Job drawing, mm, ordinate dimensions from the low corner. One solid piece. Give positions to 0.01 mm unless a question says otherwise; leave off trailing zeros. Loops run counter-clockwise (first coordinate to the right, second up) from the corner with the lowest first, then second, coordinate; pieces in that order, holes last. Notation, with made-up numbers: (15.5, 28) - (66.5, 28) arc R21 ccw to (66.5, 36) - close; hole circle Ø8 at (39.25, 80.5). An arc over 180 degrees is marked (long way). Answer as CSV lines item,"result". Start each with the question number.
Item 1: Saw through at D-D on z = 1.75. Give the cut face in (x, y), plus the area to 3 significant figures.
Item 2: Saw through at A-A on z = 9. Give the cut face in (x, y).
Item 3: Saw through at B-B on y = 1.65. State how many separate pieces and enclosed holes the cut face has, plus the area to 3 significant figures.
Item 4: Pull direction X, two halves, no side cores. Call the marked faces 1, 2 and 3: pulls with the +X half, pulls with the -X half, needs draft (parallel to the pull), parting line crosses it, or undercut.
Item 5: Pin check, flat tips, straight feed: pin 1 (1.4 mm diameter, centred on x = 5.47, z = 4.15, fed in from -Y); pin 2 (1 mm diameter, centred on x = 10, y = 0.5, fed in from -Z); pin 3 (1 mm diameter, centred on y = 1, z = 10, fed in from +X). Stop position of each tip, or through.
Item 6: Drill centre lines: L1, parallel to Z at x = 10.5, y = 0.25 (1 decimal); L2, parallel to Z at x = 4, y = 0.4 (1 decimal); L3, parallel to Z at x = 9.25, y = 0.7 (1 decimal). Where is each one in solid material? Low to high. Write a range as from..to.
Item 7: Saw through at C-C on z = 15. Give the cut face in (x, y), plus the area to 3 significant figures.
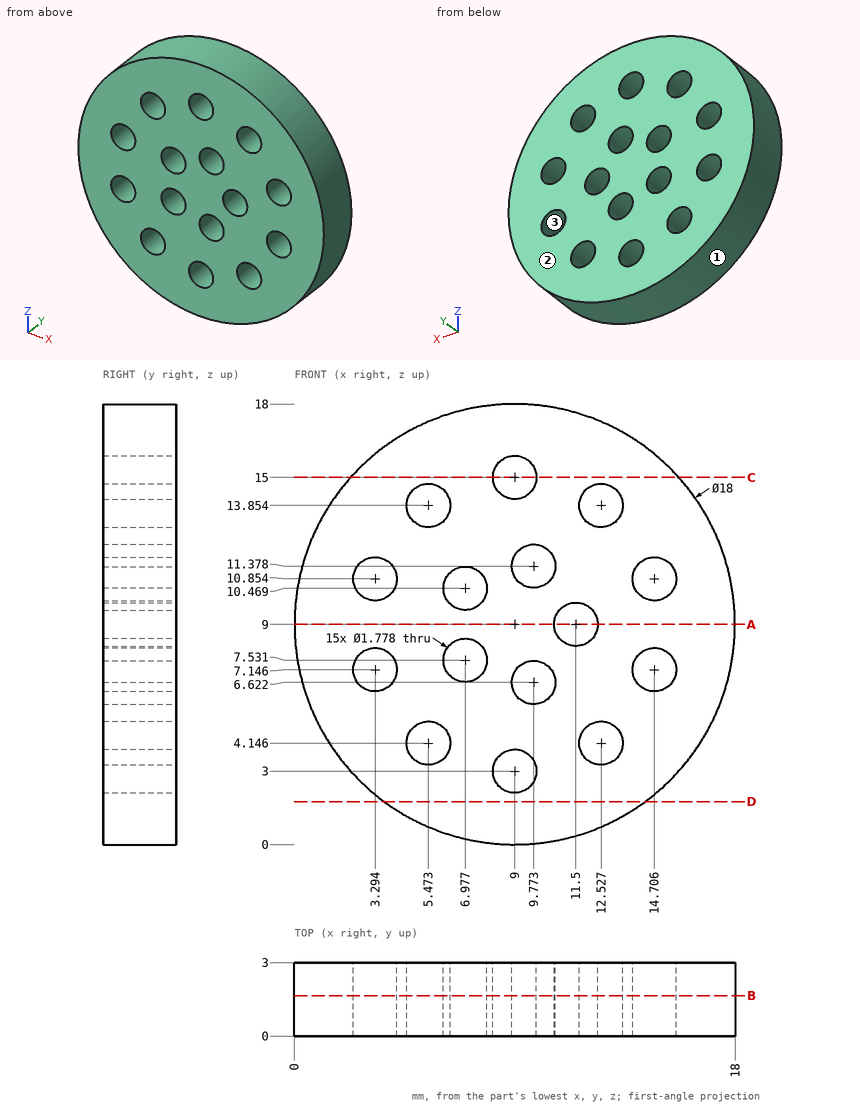
Responses:
1,outline,"(3.67, 0) - (14.33, 0) - (14.33, 3) - (3.67, 3) - close"
1,area,"32.0 mm2"
2,outline,"(0, 0) - (10.61, 0) - (10.61, 3) - (0, 3) - close; (12.39, 0) - (18, 0) - (18, 3) - (12.39, 3) - close"
3,separate pieces,"1"
3,enclosed holes,"15"
3,area,"217 mm2"
4,face 1,"parting line crosses it"
4,face 2,"needs draft"
4,face 3,"undercut"
5,pin 1,"through"
5,pin 2,"z = 0.01"
5,pin 3,"x = 17.99"
6,L1,"0.1..6.1, 7.1..10.9, 11.9..17.9"
6,L2,"1.5..6.6, 7.7..10.3, 11.4..16.5"
6,L3,"0..2.1, 3.9..5.9, 7.3..10.7, 12.1..14.1, 15.9..18"
7,outline,"(2.29, 0) - (8.11, 0) - (8.11, 3) - (2.29, 3) - close; (9.89, 0) - (15.71, 0) - (15.71, 3) - (9.89, 3) - close"
7,area,"34.9 mm2"
